from build123d import *

# Parameters (mm, degrees)
SKETCH1_W           = 40.2
SKETCH1_H           = 20
BOSS_EXTRUDE1_DEPTH = 40.5
SKETCH2_W           = 18
SKETCH2_H           = 2
BOSS_EXTRUDE2_DEPTH = 7.05
SKETCH5_R           = 3
CUT_EXTRUDE1_DEPTH  = 7.05
MIRROR2_START       = 28.5
MIRROR2_DEPTH       = 4
FILLET2_R           = 0.75
BOSS_EXTRUDE3_DEPTH = 3.5


# Read off the part's stored shape, not the designer's step: Mirror2
with BuildPart() as part:
    # Sketch1 → Boss-Extrude1 (new body)
    with BuildSketch(Plane(origin=(0, 0, 0), x_dir=(1, 0, 0), z_dir=(0, 1, 0))):
        Rectangle(SKETCH1_W, SKETCH1_H)
    extrude(amount=BOSS_EXTRUDE1_DEPTH)

    # Sketch2 → Boss-Extrude2 (add)
    with BuildSketch(Plane(origin=(20.1, 0, 0), x_dir=(0, 0, -1), z_dir=(1, 0, 0))):
        with Locations((0, 29.5)):
            Rectangle(SKETCH2_W, SKETCH2_H)
    extrude(amount=BOSS_EXTRUDE2_DEPTH)

    # Sketch5 → Cut-Extrude1 (cut)
    with BuildSketch(Plane(origin=(0, 30.5, 0), x_dir=(1, 0, 0), z_dir=(0, 1, 0))):
        with Locations((24.75, 4.95)):
            Circle(SKETCH5_R)
        with Locations((24.75, -4.95)):
            Circle(SKETCH5_R)
    extrude(amount=-CUT_EXTRUDE1_DEPTH, mode=Mode.SUBTRACT)

    # Mirror2 outline → Mirror2 (add)
    with BuildSketch(Plane(origin=(0, 0, 0), x_dir=(1, 0, 0), z_dir=(0, 1, 0)).offset(MIRROR2_START)):
        with BuildLine():
            Line((-27.15, 3.15), (-27.15, -3.15))
            ThreePointArc((-27.15, -3.15), (-21.75, -4.95), (-27.15, -6.75))
            Line((-27.15, -6.75), (-27.15, -9))
            Line((-27.15, -9), (-20.1, -9))
            Line((-20.1, -9), (-20.1, 9))
            Line((-20.1, 9), (-27.15, 9))
            Line((-27.15, 9), (-27.15, 6.75))
            ThreePointArc((-27.15, 6.75), (-21.75, 4.95), (-27.15, 3.15))
        make_face()
        with BuildLine():
            Line((27.15, 6.75), (27.15, 9))
            Line((27.15, 9), (20.1, 9))
            Line((20.1, 9), (20.1, -9))
            Line((20.1, -9), (27.15, -9))
            Line((27.15, -9), (27.15, -6.75))
            ThreePointArc((27.15, -6.75), (21.75, -4.95), (27.15, -3.15))
            Line((27.15, -3.15), (27.15, 3.15))
            ThreePointArc((27.15, 3.15), (21.75, 4.95), (27.15, 6.75))
        make_face()
    extrude(amount=MIRROR2_DEPTH)

    # Fillet2
    fillet2_edges = [part.edges().sort_by_distance(p)[0] for p in [
        (27.15, 30.5, 9),
        (27.15, 30.5, -9),
        (-27.15, 30.5, 9),
        (-27.15, 30.5, -9),
        (20.1, 20.25, 10),
        (-20.1, 20.25, 10),
        (-20.1, 20.25, -10),
        (20.1, 20.25, -10),
    ]]
    fillet(fillet2_edges, radius=FILLET2_R)

    # Sketch6 → Boss-Extrude3 (add)
    with BuildSketch(Plane(origin=(0, 40.5, 0), x_dir=(1, 0, 0), z_dir=(0, 1, 0))):
        Polygon((-9.266364833, 2.857320325), (-9.046549886, 2.408140097), (-8.578826661, 2.585104706), (-8.477624186, 2.095370547), (-7.980586038, 2.150457451), (-8.004354957, 1.650941158), (-7.50923262, 1.580689045), (-7.656479445, 1.102777065), (-7.194383277, 0.911600133), (-7.455855949, 0.485321434), (-7.055821151, 0.185232033), (-7.41509038, -0.162628729), (-7.10225261, -0.552774878), (-7.536744189, -0.80036033), (-7.330760195, -1.25604891), (-7.81317342, -1.387802348), (-7.726985934, -1.88040077), (-8.227009008, -1.888043641), (-8.266033506, -2.386600133), (-8.75224814, -2.269652207), (-8.91403257, -2.742840633), (-9.355888111, -2.508650179), (-9.630266961, -2.926738369), (-10, -2.590020434), (-10.369733039, -2.926738369), (-10.644111889, -2.508650179), (-11.08596743, -2.742840633), (-11.24775186, -2.269652207), (-11.733966494, -2.386600133), (-11.772990992, -1.888043641), (-12.273014066, -1.88040077), (-12.18682658, -1.387802348), (-12.669239805, -1.25604891), (-12.463255811, -0.80036033), (-12.89774739, -0.552774878), (-12.58490962, -0.162628729), (-12.944178849, 0.185232033), (-12.544144051, 0.485321434), (-12.805616723, 0.911600133), (-12.343520555, 1.102777065), (-12.49076738, 1.580689045), (-11.995645043, 1.650941158), (-12.019413962, 2.150457451), (-11.522375814, 2.095370547), (-11.421173339, 2.585104706), (-10.953450114, 2.408140097), (-10.733635167, 2.857320325), (-10.324615636, 2.569597349), (-10, 2.95), (-9.675384364, 2.569597349), align=None)
    extrude(amount=BOSS_EXTRUDE3_DEPTH)


solid = part.part
Geometry: final body of the model. Coordinates: model frame, mm. A direction names the side the tool comes from. Give positions to 0.01 mm unless a question says otherwise; leave off trailing zeros. Order: outer loops, then holes, each group sorted by start corner. A loop starts at its lowest first (then second) coordinate and runs counter-clockwise, first axis right, second up. Notation, with made-up numbers: (13, 31) -> (35, 31) arc R35 cw to (35, 64) -> close; hole circle Ø4 at (62, 72.25). An arc over 180 degrees is marked (long way). Answer as a JSON object with one key per item and string values.
Q1. Section B-B (y = 9). Output: boundary loops of the cut face in (x, z).
Entries:
{"outline": "(-20.1, -9.25) arc R0.75 ccw to (-19.35, -10) -> (19.35, -10) arc R0.75 ccw to (20.1, -9.25) -> (20.1, 9.25) arc R0.75 ccw to (19.35, 10) -> (-19.35, 10) arc R0.75 ccw to (-20.1, 9.25) -> close"}
Q2. Access query for faces 1 (the flat face through (23, 28.5, 0)), 2 (the flat face through (23, 32.5, 0)), 3 (the flat face through (23, 30, 9)), 4 (the flat face through (23, 30, -9)). Directions: +Z, -Z, +X, -X, +Y, -Y. A direction counts if a zero-diameter tool reaches every point of the face in a straight line with its end or side. Return the directions, or none.
Entries:
{"face 1": "+Z, -Z, +X, -Y", "face 2": "+Z, -Z, +X, +Y", "face 3": "+Z, +X, +Y, -Y", "face 4": "-Z, +X, +Y, -Y"}
Q3. Draft query along Z for faces 5 (the flat face through (-27.15, 30, 7)), 6 (the flat face through (0, 20, 10)), 7 (the cylindrical face through (-21.75, 30.47, 4.85)). Return one class per face: released by +Z, released by -Z, zero draft, split by the parting line, or undercut.
Entries:
{"face 5": "zero draft", "face 6": "released by +Z", "face 7": "undercut"}
Q4. Section A-A (x = -24.75). Output: boundary loops of the cut face in (y, z).
Entries:
{"outline": "(28.5, -9) -> (32.5, -9) -> (32.5, -7.95) -> (28.5, -7.95) -> close; (28.5, -1.95) -> (32.5, -1.95) -> (32.5, 1.95) -> (28.5, 1.95) -> close; (28.5, 7.95) -> (32.5, 7.95) -> (32.5, 9) -> (28.5, 9) -> close"}
Q5. First-contact query: pin 1 (5.5 mm diameter, centred on x = 23, z = 2.5, fed in from +Y); pin 2 (4 mm diameter, centred on x = -21, z = -4.5, fed in from +Y); pin 3 (5.5 mm diameter, centred on y = 11.5, z = 2.5, fed in from +X). Flat tips, straight axial feed; report the tip coordinate or a pass-through.
Entries:
{"pin 1": "stops at y = 32.5", "pin 2": "stops at y = 40.5", "pin 3": "stops at x = 20.1"}
Q6. Section C-C (z = 4.95). Output: boundary loops of the cut face in (x, y).
Entries:
{"outline": "(-21.75, 28.5) -> (-20.1, 28.5) -> (-20.1, 0) -> (20.1, 0) -> (20.1, 28.5) -> (21.75, 28.5) -> (21.75, 32.5) -> (20.1, 32.5) -> (20.1, 40.5) -> (-20.1, 40.5) -> (-20.1, 32.5) -> (-21.75, 32.5) -> close"}
Q7. Section D-D (x = 18). Output: boundary loops of the cut face in (y, z).
Entries:
{"outline": "(0, -10) -> (40.5, -10) -> (40.5, 10) -> (0, 10) -> close"}
Q8. Material intervals for probe 1 along Z at (x, y) = (24.75, 32.15); probe 2 along Y at (x, z) = (6.5, 0.25); probe 3 along X at (y, z) = (36, -6.5), sorted ascending.
Entries:
{"probe 1": "z = -9 to -7.95, -1.95 to 1.95, 7.95 to 9", "probe 2": "y = 0 to 40.5", "probe 3": "x = -20.1 to 20.1"}
